```python
from build123d import *

# Parameters (mm, degrees)
F1_DEPTH     = 56
F3_DEPTH     = 2.5
F5_DEPTH     = 0.75
F6_SIZE      = 0.5
F7_SIZE      = 0.5
F9_DEPTH     = 7.5
F11_DEPTH    = 4
F13_DEPTH    = 30
F15_DEPTH    = 5
F16_W        = 4
F16_H        = 9
F17_DEPTH    = 9
F19_DEPTH    = 10
F20_T1_DEPTH = 25.0355339059
F20_T3_DEPTH = 10.25
F20_T5_DEPTH = 12.017766953
F21_W        = 78.4606024017
F21_H        = 2.5
F22_DEPTH    = 10
F23_R        = 2.5
F24_DEPTH    = 4
F25_R        = 3
F27_DEPTH    = 9


# Not quite as in the source:
# - a fillet or chamfer that OpenCascade refuses, or shapes differently, is made with other operations: its cross-section is extruded or revolved along the edge and cut away or added


with BuildPart() as f1:
    # F0 (on Top) → F1 (new body)
    with BuildSketch(Plane.XY):
        Polygon((-39.2303012009, -8.5), (-46.5, -8.5), (-45, 8.5), (45, 8.5), (46.5, -8.5), (39.2303012009, -8.5), (39.2303012009, -11), (49.2303012009, -11), (47.2891247303, 11), (-47.2891247303, 11), (-49.2303012009, -11), (-39.2303012009, -11), align=None)
    extrude(amount=F1_DEPTH)

    # F2 (on face) → F3 (join)
    with BuildSketch(Plane.XY.offset(56)):
        Polygon((-46.5, -8.5), (-39.2303012009, -8.5), (-37.7303012009, 8.5), (-45, 8.5), align=None)
        Polygon((46.5, -8.5), (45, 8.5), (37.7303012009, 8.5), (39.2303012009, -8.5), align=None)
    extrude(amount=-F3_DEPTH)

    # F4 (on face) → F5 (join)
    with BuildSketch(Plane(origin=(0, 0, 0), x_dir=(1, 0, 0), z_dir=(0, 0, -1))):
        Polygon((-40.7303012009, 7.75), (-40.2303012009, 8.5), (-45.5, 8.5), (-45, 7.75), align=None)
        Polygon((45, 7.75), (45.5, 8.5), (40.2303012009, 8.5), (40.7303012009, 7.75), align=None)
    extrude(amount=-F5_DEPTH)

    # F6
    f6_edges = [f1.edges().sort_by_distance(p)[0] for p in [
        (42.865151, -7.75, 0.75),
    ]]
    chamfer(f6_edges, length=F6_SIZE)

    # F7
    f7_edges = [f1.edges().sort_by_distance(p)[0] for p in [
        (-42.865151, -7.75, 0.75),
    ]]
    chamfer(f7_edges, length=F7_SIZE)

    # F8 (on face) → F9 (cut)
    with BuildSketch(Plane(origin=(0, 0, 0), x_dir=(1, 0, 0), z_dir=(0, 0, -1))):
        Polygon((-46.7205882353, 11), (-46.5, 8.5), (-45.8406183737, 8.5), (-46.061206609, 11), align=None)
        Polygon((46.5, 8.5), (46.7205882353, 11), (46.061206609, 11), (45.8406183737, 8.5), align=None)
    extrude(amount=-F9_DEPTH, mode=Mode.SUBTRACT)

    # F10 (on face) → F11 (join)
    with BuildSketch(Plane.XY.offset(56)):
        Polygon((-74.2303012009, -7), (-74.2303012009, -11), (-74.2303012009, -41), (-39.2303012009, -41), (-39.2303012009, -11), (-49.2303012009, -11), (-48.8773600244, -7), align=None)
        Polygon((49.2303012009, -11), (39.2303012009, -11), (39.2303012009, -20), (58.2303012009, -20), (58.2303012009, -11), (58.2303012009, -7), (48.8773600244, -7), align=None)
    extrude(amount=-F11_DEPTH)

    # F12 (on face) → F13 (join)
    with BuildSketch(Plane(origin=(0, 0, 52), x_dir=(1, 0, 0), z_dir=(0, 0, -1))):
        Polygon((-74.2303012009, 7), (-48.8773600244, 7), (-49.2303012009, 11), (-74.2303012009, 11), align=None)
    extrude(amount=F13_DEPTH)

    # F14 (on face) → F15 (join)
    with BuildSketch(Plane(origin=(0, 0, 52), x_dir=(1, 0, 0), z_dir=(0, 0, -1))):
        Polygon((58.2303012009, 20), (39.2303012009, 20), (39.2303012009, 11), (49.2303012009, 11), (48.8773600244, 7), (58.2303012009, 7), align=None)
    extrude(amount=F15_DEPTH)

    # F16 (on face) → F17 (cut)
    with BuildSketch(Plane.YZ.offset(58.2303012009)):
        Polygon((-11, 47), (-20, 56), (-20, 47), align=None)
        with Locations((-9, 51.5)):
            Rectangle(F16_W, F16_H)
    extrude(amount=-F17_DEPTH, mode=Mode.SUBTRACT)

    # F18 (on face) → F19 (cut)
    with BuildSketch(Plane.YZ.offset(49.2303012009)):
        Polygon((-11, 47), (-20, 56), (-20, 47), align=None)
    extrude(amount=-F19_DEPTH, mode=Mode.SUBTRACT)

    # F20: fillet of radius 0.5 on 3 edges, made by hand

    # F20_s2 → F20_t1 (cut)
    with BuildSketch(Plane.YZ.offset(36.2125342479)):
        with BuildLine():
            ThreePointArc((-19.1464466094, 55.1464466094), (-19.2548329851, 55.6913417162), (-18.7928932188, 56))
            Line((-18.7928932188, 56), (-20, 56))
            Line((-20, 56), (-19.1464466094, 55.1464466094))
        make_face()
    extrude(amount=F20_T1_DEPTH, mode=Mode.SUBTRACT)

    # F20_s4 → F20_t3 (cut)
    with BuildSketch(Plane.YZ.offset(49.2303012009)):
        with BuildLine():
            ThreePointArc((-11, 55.5), (-11.1464466094, 55.8535533906), (-11.5, 56))
            Line((-11.5, 56), (-11, 56))
            Line((-11, 56), (-11, 55.5))
        make_face()
    extrude(amount=F20_T3_DEPTH, mode=Mode.SUBTRACT)

    # F20_s6 → F20_t5 (cut)
    with BuildSketch(Plane.YZ.offset(49.2303012009)):
        with BuildLine():
            ThreePointArc((-11.8535533906, 47.8535533906), (-11.3086582838, 47.7451670149), (-11, 48.2071067812))
            Line((-11, 48.2071067812), (-11, 47))
            Line((-11, 47), (-11.8535533906, 47.8535533906))
        make_face()
    extrude(amount=F20_T5_DEPTH, mode=Mode.SUBTRACT)

    # F21 (on face) → F22 (join)
    with BuildSketch(Plane.XY.offset(56)):
        with Locations((0, -9.75)):
            Rectangle(F21_W, F21_H)
    extrude(amount=-F22_DEPTH)

    # F23 (on face) → F24 (cut)
    with BuildSketch(Plane.XY.offset(56)):
        with Locations((-70.7696987991, -32)):
            Circle(F23_R)
    extrude(amount=-F24_DEPTH, mode=Mode.SUBTRACT)

    # F25
    f25_edges = [f1.edges().sort_by_distance(p)[0] for p in [
        (-74.230301, -41, 54),
        (-39.230301, -41, 54),
        (-74.230301, -9, 22),
        (-49.053831, -9, 22),
        (-39.230301, -11, 54),
    ]]
    fillet(f25_edges, radius=F25_R)

    # F26 (on face) → F27 (cut)
    with BuildSketch(Plane.YZ.offset(58.2303012009)):
        Polygon((-11, 52), (-11, 56), (-20, 56), (-16, 52), align=None)
    extrude(amount=-F27_DEPTH, mode=Mode.SUBTRACT)


solid = f1.part
```
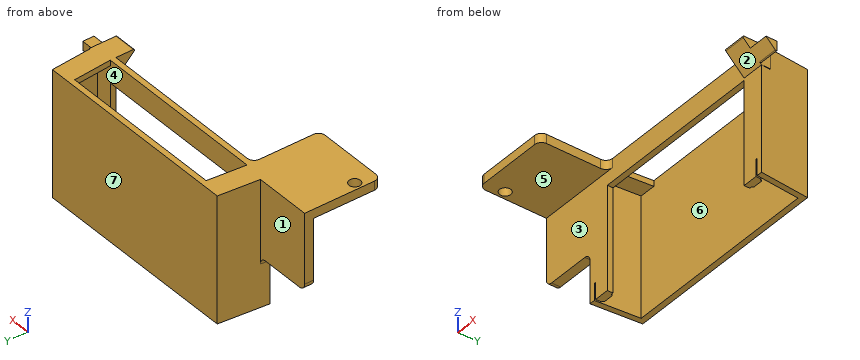
Build history of the part. All positions in model axes, mm. Face numbers are marked on the shaded views. A direction names the side the tool comes from. Give positions to 0.01 mm unless a question says otherwise; leave off trailing zeros. Loops run counter-clockwise (first coordinate to the right, second up) from the corner with the lowest first, then second, coordinate; pieces in that order, holes last.
Item 1: Slice it at A-A, the plane y = -32. List the corners of the cut face in (x, z).
Answers follow:
outline: (-74.23, 52) - (-73.27, 52) - (-73.27, 56) - (-74.23, 56) - close; (-68.27, 52) - (-39.23, 52) - (-39.23, 56) - (-68.27, 56) - close
Item 2: Slice it at C-C, the plane x = -4. List the corners of the cut face in (y, z).
Answers follow:
outline: (-11, 46) - (-8.5, 46) - (-8.5, 56) - (-11, 56) - close; (8.5, 0) - (11, 0) - (11, 56) - (8.5, 56) - close
Item 3: Slice it at D-D, the plane y = -1.5. List the corners of the cut face in (x, z), and give its area (3 significant figures).
Answers follow:
outline: (-48.39, 0) - (-45.88, 0) - (-45.88, 53.5) - (-38.61, 53.5) - (-38.61, 56) - (-48.39, 56) - close; (38.61, 53.5) - (45.88, 53.5) - (45.88, 0) - (48.39, 0) - (48.39, 56) - (38.61, 56) - close
area: 317 mm2
Item 4: Pull direction Y, two halves, no side cores. Call the marked faces 4, 5, 6 and 7: released by +Y, released by -Y, zero draft, split by the parting line, or undercut.
Answers follow:
face 4: undercut
face 5: zero draft
face 6: undercut
face 7: released by +Y
Item 5: Which spindle directions (+Z, -Z, +X, -X, +Y, -Y) get a long thin tool onto all of the face, cutting with end or side? Do the marked faces 1, 2 and 3. Say none if no direction does.
Answers follow:
face 1: +Z, -Z, -X, +Y
face 2: -Z, +X, -Y
face 3: -Z, -Y
Item 6: Drill centre lines: line 1 (Y direction, x = -15.5, z = 19.5); line 2 (Z direction, x = -62, y = -14.5); line 3 (Y direction, x = -13, z = 51.5). Where is each one in solid material? Low to high.
Answers follow:
line 1: y = 8.5 to 11
line 2: z = 52 to 56
line 3: y = -11 to -8.5, 8.5 to 11
Item 7: Flat gauge pins, fed straight in: pin 1 (1.2 mm diameter, centred on y = -10, z = 15.5, fed in from -X) (3 decimals); pin 2 (15 mm diameter, centred on x = -57, y = -26.5, fed in from -Z); pin 3 (2 mm diameter, centred on x = 32.5, z = 10.5, fed in from -Y). Where does each tip first touch, or does it go through?
Answers follow:
pin 1: stops at x = -49.195
pin 2: stops at z = 52
pin 3: stops at y = 8.5
Item 8: Slice it at B-B, the plane z = 39.5. List the corners of the cut face in (x, y), and give its area (3 significant figures).
Answers follow:
outline: (-74.23, -11) - (-39.23, -11) - (-39.23, -8.5) - (-46.5, -8.5) - (-45, 8.5) - (45, 8.5) - (46.5, -8.5) - (39.23, -8.5) - (39.23, -11) - (49.23, -11) - (47.29, 11) - (-47.29, 11) - (-48.88, -7) - (-74.23, -7) - close
area: 472 mm2
